from build123d import *

# Parameters (mm, degrees)
F1_DEPTH  = 101.6
F3_DEPTH  = 108.6532940183
F4_W      = 52.07
F4_H      = 52.07
F5_DEPTH  = 12.7
F6_R      = 3.175
F7_R      = 3.175
F10_W     = 114.2207605299
F10_H     = 103.8881577551
F11_DEPTH = 25.4


with BuildPart() as f1:
    # F0 (on Right) → F1 (new body)
    with BuildSketch(Plane.YZ):
        Polygon((95.3280799156, 185.0426944046), (-38.8999396909, 0), (62.7000603091, 0), align=None)
    extrude(amount=F1_DEPTH)

    # F2 (on face) → F3 (cut, through all)
    with BuildSketch(Plane(origin=(0, -25.4882702356, 18.4889225048), x_dir=(1, 0, 0), z_dir=(0, -0.8094606054, 0.587174189))):
        Polygon((0, 205.7589594597), (0, -22.8410405403), (50.8, 205.7589594597), align=None)
        Polygon((101.6, 205.7589594597), (50.8, 205.7589594597), (101.6, -22.8410405403), align=None)
    extrude(amount=-F3_DEPTH, mode=Mode.SUBTRACT)

    # F4 (on face) → F5 (cut)
    with BuildSketch(Plane(origin=(0, -25.4882702356, 18.4889225048), x_dir=(1, 0, 0), z_dir=(0, -0.8094606054, 0.587174189))):
        with Locations((51.483128581, 45.8012033367)):
            Rectangle(F4_W, F4_H)
    extrude(amount=-F5_DEPTH, mode=Mode.SUBTRACT)

    # F6
    f6_edges = [f1.edges().sort_by_distance(p)[0] for p in [
        (25.448129, 21.832169, 72.908943),
    ]]
    fillet(f6_edges, radius=F6_R)

    # F7
    f7_edges = [f1.edges().sort_by_distance(p)[0] for p in [
        (25.448129, -8.741991, 30.760329),
        (77.518129, -8.741991, 30.760329),
        (77.518129, 21.832169, 72.908943),
    ]]
    fillet(f7_edges, radius=F7_R)

    # F10 (on face) → F11 (cut)
    with BuildSketch(Plane(origin=(-4.6941337345, 4.3288858466, -4.5218095202), x_dir=(-0.3984565906, -0.8330111765, -0.3838290314), z_dir=(-0.5999369127, 0.5532561612, -0.5779129008))):
        with Locations((-60.2949896129, -21.5842779726)):
            Rectangle(F10_W, F10_H)
    extrude(amount=F11_DEPTH, mode=Mode.SUBTRACT)


solid = f1.part
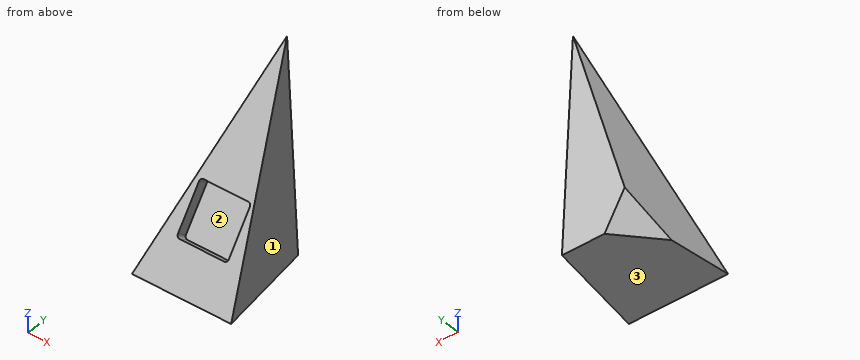
The listing builds one solid part. Answer for the finished solid, in the listing's coordinates (mm). Face numbers are marked on the shaded views. Give positions to 0.01 mm unless a question says otherwise; leave off trailing zeros. Loops run counter-clockwise (first coordinate to the right, second up) from the corner with the lowest first, then second, coordinate; pieces in that order, holes last. Notation, with made-up numbers: M -9,54 L 32,54 A26 cw 32,80 Z; hole C -3.75,72 d11. An arc over 180 degrees is marked long. Answer as CSV lines item,"result".
Item 1: Straight lines are drawn through the part: line 1 along X through (y, z) = (10, 50); line 2 along Z through (x, y) = (77, -10); line 3 along X through (y, z) = (82, 153). For each, find the intervals that lie inside material, in ascending order. Write a range as [from, to].
Values follow:
line 1,"x = [15.37, 25.45], [77.52, 86.23]"
line 2,"z = [0, 33.45]"
line 3,"x = [43.3, 58.3]"
Item 2: Given pin 1 Ø3 at (y, z) = (-6, 27.5) entering from +X; pin 2 Ø6 at (x, y) = (18, -3) entering from +Z; pin 3 Ø1 at (x, y) = (54.5, 65) entering from +Z, each flat-ended and moving along its own axis, determine where each tip first touches the part or whether it passes through.
Values follow:
pin 1,"stops at x = 92.69"
pin 2,"stops at z = 53.63"
pin 3,"stops at z = 143.92"
Item 3: The part is cut by section D-D (x = 22.5). Give the vertices of the cut face in (y, z), and give its area (3 significant figures).
Values follow:
outline,"M -38.9,0 L 38.54,0 L 67.61,27.83 L 70.73,45.56 L 20.55,81.96 Z"
area,"5,120 mm^2"
Item 4: The part is cut by section A-A (x = 40). Give the vertices of the cut face in (y, z), and give its area (3 significant figures).
Values follow:
outline,"M -38.9,0 L 57.52,0 L 63.75,5.97 L 85.94,131.81 L 66.79,145.7 L 16.69,76.64 L 26.97,69.18 L -3.6,27.03 L -13.88,34.49 Z"
area,"8,150 mm^2"
Item 5: The mould has two halves that part along Z. Classify the marked faces 1, 2 and 3: released by +Z, released by -Z, zero draft, split by the parting line, or undercut.
Values follow:
face 1,"released by +Z"
face 2,"undercut"
face 3,"released by -Z"
Item 6: The part is cut by section B-B (y = 5.5). Give the vertices of the cut face in (x, z), and give its area (3 significant figures).
Values follow:
outline,"M 5.79,0 L 95.81,0 L 84.8,61.21 L 77.52,61.21 L 77.52,39.58 L 25.45,39.58 L 25.45,61.21 L 16.8,61.21 Z"
area,"3,710 mm^2"
Item 7: The part is cut by section C-C (z = 154.5). Give the vertices of the cut face in (x, y).
Values follow:
outline,"M 42.42,73.17 L 59.18,73.17 L 57,89.94 L 44.6,89.94 Z"
